```python
from build123d import *

# Parameters (mm, degrees)
SKETCH1_R           = 1.5025
BOSS_EXTRUDE1_DEPTH = 3
SKETCH2_R           = 5
SKETCH2_R_2         = 3.5025
BOSS_EXTRUDE2_DEPTH = 3


with BuildPart() as part:
    # Sketch1 → Boss-Extrude1 (new body)
    with BuildSketch(Plane(origin=(0, 0, 0), x_dir=(1, 0, 0), z_dir=(0, 1, 0))):
        with BuildLine():
            Line((-18.4, 6), (18.4, 6))
            ThreePointArc((18.4, 6), (21.9, 0), (18.4, -6))
            Line((18.4, -6), (-18.4, -6))
            ThreePointArc((-18.4, -6), (-21.9, 0), (-18.4, 6))
        make_face()
        with Locations((10, 0)):
            Circle(SKETCH1_R, mode=Mode.SUBTRACT)
        with Locations((-10, 0)):
            Circle(SKETCH1_R, mode=Mode.SUBTRACT)
    extrude(amount=BOSS_EXTRUDE1_DEPTH)

    # Sketch2 → Boss-Extrude2 (add)
    with BuildSketch(Plane(origin=(0, 3, 0), x_dir=(1, 0, 0), z_dir=(0, 1, 0))):
        Circle(SKETCH2_R)
        Circle(SKETCH2_R_2, mode=Mode.SUBTRACT)
    extrude(amount=BOSS_EXTRUDE2_DEPTH)


solid = part.part
```
Here's how the part is built. I have some questions about the finished solid (model axes, mm). A direction names the side the tool comes from. Give positions to 0.01 mm unless a question says otherwise; leave off trailing zeros. Loops run counter-clockwise (first coordinate to the right, second up) from the corner with the lowest first, then second, coordinate; pieces in that order, holes last. Notation, with made-up numbers: M 8,-13 L 39,-13 A6 ccw 39,-3 Z; hole C -21.5,-37 d7. An arc over 180 degrees is marked long. Return JSON: item names as keys, results as strings.
Item 1: Thinking about a two-plate mould opening in X: for faces 3 (the flat face through (0, 1, -6)), 4 (the cylindrical face through (-11.5, 1.5, -0.1)), 5 (the cylindrical face through (21.9, 1.5, -0.1)), which applies, released by +X, released by -X, zero draft, split by the parting line, or undercut?
A:
{"face 3": "zero draft", "face 4": "undercut", "face 5": "released by +X"}
Item 2: Imagine slicing it at A-A on x = 10. List the corners of the cut face in (y, z) for me.
A:
{"outline": "M 0,-6 L 3,-6 L 3,-1.5 L 0,-1.5 Z; M 0,1.5 L 3,1.5 L 3,6 L 0,6 Z"}
Item 3: Imagine slicing it at C-C on y = 1.1. List the corners of the cut face in (x, z) for me (1 decimal).
A:
{"outline": "M -18.4,-6 L 18.4,-6 A6.9 ccw 18.4,6 L -18.4,6 A6.9 ccw Z; hole C -10,0 d3; hole C 10,0 d3"}
Item 4: Imagine slicing it at B-B on z = 0. List the corners of the cut face in (x, y) for me.
A:
{"outline": "M -21.9,0 L -11.5,0 L -11.5,3 L -21.9,3 Z; M -8.5,0 L 8.5,0 L 8.5,3 L 5,3 L 5,6 L 3.5,6 L 3.5,3 L -3.5,3 L -3.5,6 L -5,6 L -5,3 L -8.5,3 Z; M 11.5,0 L 21.9,0 L 21.9,3 L 11.5,3 Z"}
Item 5: Imagine slicing it at D-D on x = 0. List the corners of the cut face in (y, z) for me.
A:
{"outline": "M 0,-6 L 3,-6 L 3,-5 L 6,-5 L 6,-3.5 L 3,-3.5 L 3,3.5 L 6,3.5 L 6,5 L 3,5 L 3,6 L 0,6 Z"}
Item 6: Please list where these lines run through material, in increasing order: line 1 (X direction, y = 1.25, z = 0); line 2 (X direction, y = 4.1, z = 0); line 3 (X direction, y = 2.15, z = 1).
A:
{"line 1": "x = -21.9 to -11.5, -8.5 to 8.5, 11.5 to 21.9", "line 2": "x = -5 to -3.5, 3.5 to 5", "line 3": "x = -21.83 to -11.12, -8.88 to 8.88, 11.12 to 21.83"}
Item 7: On a 3-axis mill with a long thin cutter (end or side, diameter ignored), from which of +Z, -Z, +X, -X, +Y, -Y can I reach the whole of each face in a straight line? I mean faces 1 (the cylindrical face through (-0.76, 4.48, 3.42)), 2 (the flat face through (0, 0, 0)). Say none if no direction works.
A:
{"face 1": "+Y", "face 2": "+Z, -Z, +X, -X, -Y"}
Item 8: I'm going to push a flat-ended pin straight in: pin 1 Ø6 at (x, z) = (15, 1) entering from +Y. Where does the tip first touch, or does it pass through?
A:
{"pin 1": "stops at y = 3"}
